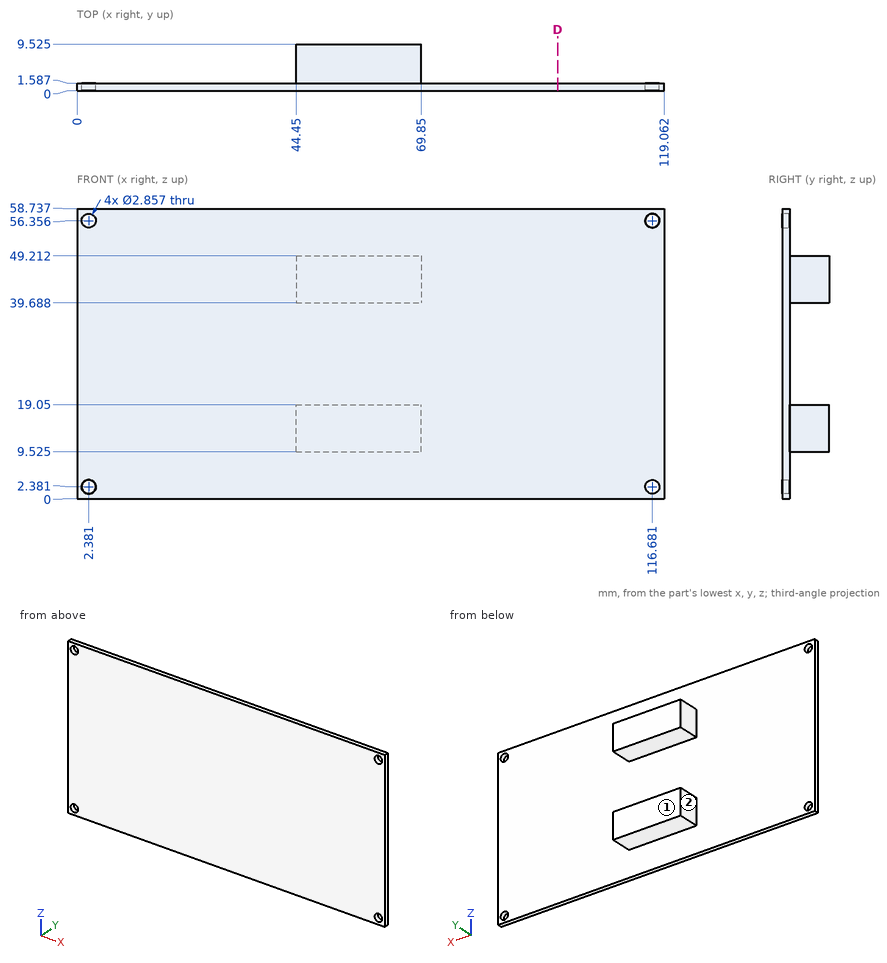
Study the drawing (mm; zero at the part's minimum x, y, z) and answer. A direction names the side the tool comes from. Give positions to 0.01 mm unless a question says otherwise; leave off trailing zeros. Loops run counter-clockwise (first coordinate to the right, second up) from the corner with the lowest first, then second, coordinate; pieces in that order, holes last. Notation, with made-up numbers: M 9.5,36 L 31.5,36 A17 cw 31.5,42 Z; hole C -5.5,-18 d8. An arc over 180 degrees is marked long. Use CSV: the item, a comma, the result in double quotes.
1) Given P1, Ø4, axis at x = 77, z = 24, coming from the +Y side; P2, Ø2.5, axis at x = 53, y = 4, coming from the +Z side; P3, Ø2.5, axis at y = 7, z = 16.5, coming from the -X side, each flat-ended and moving along its own axis, determine where each tip first touches the part or whether it passes through.
Answer:
P1,"y = 1.59"
P2,"z = 49.21"
P3,"x = 44.45"
2) Consider L1, parallel to Y at x = 114.5, z = 9.5; L2, parallel to X at y = 8, z = 19. Determine where each line is inside the solid, lowest interval first.
Answer:
L1,"0 to 1.59"
L2,"44.45 to 69.85"
3) Find section D-D on x = 97.5. Write down the section's boundary in (y, z).
Answer:
outline,"M 0,0 L 1.59,0 L 1.59,58.74 L 0,58.74 Z"
4) Which of the six approach directions +Z, -Z, +X, -X, +Y, -Y give full straight-line access (tool end or side, diameter ignored) to the marked faces 1 and 2?
Answer:
face 1,"+Z, -Z, +X, -X, +Y"
face 2,"+Z, -Z, -X, +Y"
